Answer from the drawing. Dimensions are ordinates in mm from the lowest x, y and z of the part. A direction names the side the tool comes from. Coordinates: 2 decimals unless noted, no trailing zeros. Order: outer loops, then holes, each group sorted by start corner. A loop starts at its lowest first (then second) coordinate and runs counter-clockwise, first axis right, second up. Notation, with made-up numbers: (55.25, 83.25) -> (84.25, 83.25) arc R30 ccw to (84.25, 114.25) -> close; hole circle Ø6 at (63.5, 29.5). An arc over 180 degrees is marked (long way). Answer in a Markdown table with one row per item.
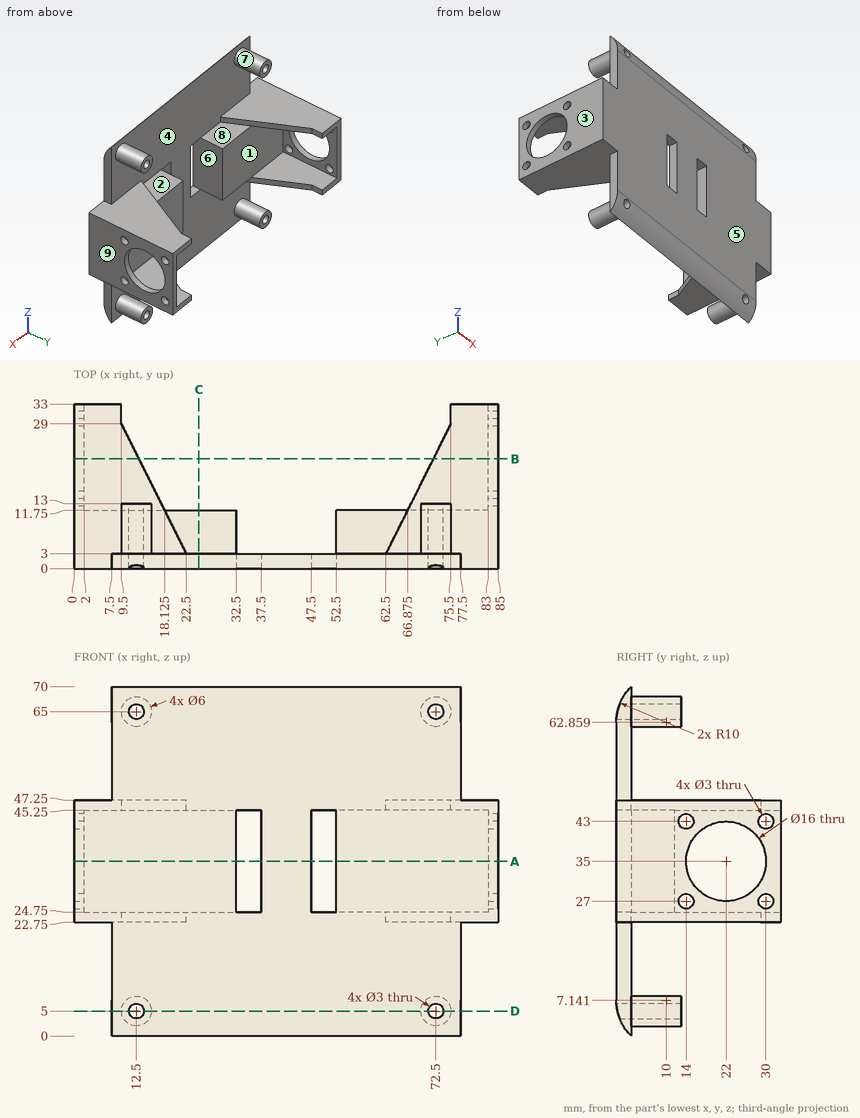
(1) Flat-ended cylindrical pins translate along their axes: pin 1 (8 mm diameter, centred on x = 64.5, y = 14.5, fed in from -Z); pin 2 (22.5 mm diameter, centred on x = 18, z = 38, fed in from +Y); pin 3 (12 mm diameter, centred on x = 36, y = 7.5, fed in from +Z); pin 4 (3.5 mm diameter, centred on x = 49, y = 1.5, fed in from -Z). Find the tip coordinate at first contact, or state that the pin passes through.
Check values:
| item | result |
|---|---|
| pin 1 | z = 22.75 |
| pin 2 | y = 33 |
| pin 3 | z = 70 |
| pin 4 | z = 0 |
(2) Find the intervals of material crossed by line 1 along X through (y, z) = (9, 65); line 2 along Z through (x, y) = (72.5, 7); line 3 along X through (y, z) = (13.5, 32), in increasing order. Write a range as from..to.
Check values:
| item | result |
|---|---|
| line 1 | 9.5..11, 14..15.5, 69.5..71, 74..75.5 |
| line 2 | 2..3.5, 6.5..8, 22.75..47.25, 62..63.5, 66.5..68 |
| line 3 | 0..2, 83..85 |
(3) A cutting plane is placed at B-B, the plane y = 22. Determine the outline of the cut face in (x, z).
Check values:
| item | result |
|---|---|
| outline | (0, 22.75) -> (13, 22.75) -> (13, 24.75) -> (2, 24.75) -> (2, 27) -> (0, 27) -> close; (0, 43) -> (2, 43) -> (2, 45.25) -> (13, 45.25) -> (13, 47.25) -> (0, 47.25) -> close; (72, 22.75) -> (85, 22.75) -> (85, 27) -> (83, 27) -> (83, 24.75) -> (72, 24.75) -> close; (72, 45.25) -> (83, 45.25) -> (83, 43) -> (85, 43) -> (85, 47.25) -> (72, 47.25) -> close |
(4) For a pull along Z with two mould halves and no side action, classify the marked faces 1, 2, 3 and 4 as released by +Z, released by -Z, zero draft, split by the parting line, or undercut.
Check values:
| item | result |
|---|---|
| face 1 | undercut |
| face 2 | released by +Z |
| face 3 | zero draft |
| face 4 | undercut |
(5) A cutting plane is placed at A-A, the plane z = 35. Determine the outline of the cut face in (x, y), then the cut area to 3 significant figures.
Check values:
| item | result |
|---|---|
| outline | (0, 0) -> (32.5, 0) -> (32.5, 11.75) -> (2, 11.75) -> (2, 14) -> (0, 14) -> close; (0, 30) -> (2, 30) -> (2, 33) -> (0, 33) -> close; (37.5, 0) -> (47.5, 0) -> (47.5, 3) -> (37.5, 3) -> close; (52.5, 0) -> (85, 0) -> (85, 14) -> (83, 14) -> (83, 11.75) -> (52.5, 11.75) -> close; (83, 30) -> (85, 30) -> (85, 33) -> (83, 33) -> close |
| area | 815 mm² |
(6) Which of the six approach directions +Z, -Z, +X, -X, +Y, -Y give full straight-line access (tool end or side, diameter ignored) to the marked faces 5, 6, 7, 8 and 9?
Check values:
| item | result |
|---|---|
| face 5 | +Z, -Z, +X, -X, -Y |
| face 6 | +Y, -Y |
| face 7 | +Y |
| face 8 | +Z, +Y |
| face 9 | +Z, -Z, +X, +Y, -Y |
(7) A cutting plane is placed at D-D, the plane z = 5. Determine the outline of the cut face in (x, y), then the cut area to 3 significant figures.
Check values:
| item | result |
|---|---|
| outline | (7.5, 0.23) -> (11, 0.23) -> (11, 13) -> (9.5, 13) -> (9.5, 3) -> (7.5, 3) -> close; (14, 0.23) -> (71, 0.23) -> (71, 13) -> (69.5, 13) -> (69.5, 3) -> (15.5, 3) -> (15.5, 13) -> (14, 13) -> close; (74, 0.23) -> (77.5, 0.23) -> (77.5, 3) -> (75.5, 3) -> (75.5, 13) -> (74, 13) -> close |
| area | 237 mm² |
(8) A cutting plane is placed at C-C, the plane x = 25. Determine the outline of the cut face in (y, z).
Check values:
| item | result |
|---|---|
| outline | (0, 7.14) arc R10 ccw to (3, 0) -> (3, 24.75) -> (11.75, 24.75) -> (11.75, 45.25) -> (3, 45.25) -> (3, 70) arc R10 ccw to (0, 62.86) -> close |
